Here's how the part is built. I have some questions about the finished solid (model axes, mm). A direction names the side the tool comes from. Round coordinates to 2 decimals unless told otherwise and drop trailing zeros. Order: outer loops, then holes, each group sorted by start corner. A loop starts at its lowest first (then second) coordinate and runs counter-clockwise, first axis right, second up. Notation, with made-up numbers: M 19.25,66.25 L 61.25,66.25 A31 cw 61.25,95.25 Z; hole C -28,-33.75 d8. An arc over 180 degrees is marked long. Write item = value, one per line. Start each with the question number.
Item 1: I'm going to push flat-ended pins straight in: P1, Ø4, axis at x = 10, z = 0, coming from the +Y side; P2, Ø8, axis at x = 11.5, y = -6.5, coming from the -Z side; P3, Ø5, axis at x = 4.5, z = -11, coming from the -Y side. Where does each tip first touch, or does it pass through?
Item 2: For faces 4 (the face through (7, -11, 0)), 5 (the face through (-2, -15, 15)), 6 (the face through (7, 0, 9)), 7 (the face through (7, 0, 11)), 8 (the face through (-3, 0, 0)), which set-ups out of +Z, -Z, +X, -X, +Y, -Y let a thin tool reach every point of the face, with its end or its side?
Item 3: I want a section at A-A, the plane x = 10. List the corners of the cut face in (y, z) for me, plus the area to 3 significant figures.
Item 4: We'd pull the mould along X, two halves only. Please class faces 1 (the face through (7, 0, -11)), 2 (the face through (0, 14, 0)), 3 (the face through (9.63, -9.99, 1.66)): pulls with the +X half, pulls with the -X half, needs draft (parallel to the pull), parting line crosses it, or undercut.
Item 5: I want a section at B-B, the plane z = 16. List the corners of the cut face in (x, y) for me, plus the area to 3 significant figures.
Item 6: I want a section at D-D, the plane y = 0. List the corners of the cut face in (x, z) for me.
Item 7: Please list where these lines run through material, in increasing order: L1, parallel to Z at x = 4.75, y = 6; L2, parallel to Z at x = 10, y = 9.5.
Item 8: I want a section at C-C, the plane x = 5. List the corners of the cut face in (y, z) for me.
Autodesk Inventor part; units mm, degrees
ref_plane "YZ Plane" through (0, 0, 0) normal (1, 0, 0) x (0, 1, 0)
ref_plane "XZ Plane" through (0, 0, 0) normal (0, 1, 0) x (-1, 0, 0)
ref_plane "XY Plane" through (0, 0, 0) normal (0, 0, 1) x (1, 0, 0)
sketch "スケッチ1" plane through (0, 0, 0) normal (1, 0, 0) x (0, 1, 0)
  line L0 (9, -9) -> (-9, -9)
  line L1 (-9, -9) -> (-9, 9)
  line L2 (-9, 9) -> (9, 9)
  line L3 (9, 9) -> (9, -9)
  line L4 (9, -9) -> (-9, 9) construction
  line L5 (-9, -9) -> (9, 9) construction
  line L6 (11, -11) -> (-11, -11)
  line L7 (-11, -11) -> (-11, 11)
  line L8 (-11, 11) -> (11, 11)
  line L9 (11, 11) -> (11, -11)
  line L10 (11, -11) -> (-11, 11) construction
  line L11 (-11, -11) -> (11, 11) construction
  point P0 (0, 0)
  dimension "d0" = 18
  dimension "d1" = 18
  dimension "d2" = 22
  dimension "d3" = 22
extrude "押し出し1" add sketch "スケッチ1" along normal blind 15
sketch "スケッチ2" plane through (0, -11, 11) normal (0, 0, 1) x (1, 0, 0)
  circle A0 centre (10, 11) radius 1.7
  point P0 (0, 11)
  dimension "d6" = 3.4
extrude "押し出し2" cut sketch "スケッチ2" against normal blind 30
sketch "スケッチ3" plane through (0, 11, 11) normal (0, 1, 0) x (1, 0, 0)
  circle A0 centre (10, 11) radius 1.7
  point P0 (0, 11)
  dimension "d9" = 3.4
extrude "押し出し3" cut sketch "スケッチ3" against normal blind 30
sketch "スケッチ4" plane through (0, 0, 0) normal (-1, 0, 0) x (0, 0, 1)
  line L0 (20, -20) -> (-20, -20)
  line L1 (-20, -20) -> (-20, 20)
  line L2 (-20, 20) -> (20, 20)
  line L3 (20, 20) -> (20, -20)
  line L4 (20, -20) -> (-20, 20) construction
  line L5 (-20, -20) -> (20, 20) construction
  point P0 (0, 0)
  dimension "d12" = 40
  dimension "d13" = 40
extrude "押し出し4" add sketch "スケッチ4" along normal blind 3
sketch "スケッチ5" plane through (-3, 0, 0) normal (-1, 0, 0) x (0, 0, 1)
  circle A0 centre (16, 0) radius 2.25
  circle A1 centre (-16, 0) radius 2.25
  point P0 (0, 0)
  dimension "d16" = 4.5
  dimension "d17" = 4.5
extrude "押し出し5" cut sketch "スケッチ5" against normal blind 3
sketch "スケッチ6" plane through (-3, 0, 0) normal (-1, 0, 0) x (0, 0, 1)
  line L0 (20, 20) -> (-20, 20)
  line L1 (10, 20) -> (20, 10)
  line L2 (20, -20) -> (20, 20)
  line L3 (10, 20) -> (24.1421, 20) construction
  line L4 (20, 10) -> (20, 20)
  line L5 (20, 20) -> (10, 20)
  line L6 (-20, -20) -> (20, -20)
  line L7 (20, -20) -> (10, -20)
  line L8 (10, -20) -> (20, -10)
  line L9 (20, -10) -> (20, -20)
  line L10 (-20, 20) -> (-20, -20)
  line L11 (-20, -20) -> (-10, -20)
  line L12 (-10, -20) -> (-20, -10)
  line L13 (-20, -10) -> (-20, -20)
  line L14 (-20, 20) -> (-10, 20)
  line L15 (-10, 20) -> (-20, 10)
  line L16 (-20, 10) -> (-20, 20)
  point P0 (0, 0)
  dimension "d20" = 45
  dimension "d21" = 10
  dimension "d22" = 45
  dimension "d23" = 10
  dimension "d24" = 45
  dimension "d25" = 10
  dimension "d26" = 45
extrude "押し出し6" cut sketch "スケッチ6" against normal blind 3 contours L2 L1 L0 | L15 L10 L0 | L2 L6 L8 | L12 L6 L10
properties part number "square_ber_holder" material "ABS プラスチック"
Filled in:
q1.P1 = 11
q1.P2 = -11
q1.P3 = -11
q2.face_4 = +Z, -Z, +X, -Y
q2.face_5 = +Z, +X, -X, -Y
q2.face_6 = +X
q2.face_7 = +Z, +X, +Y, -Y
q2.face_8 = +Z, -Z, -X, +Y, -Y
q3.outline = M -11,-11 L -1.7,-11 L -1.7,-9 L -9,-9 L -9,-1.7 L -11,-1.7 Z; M -11,1.7 L -9,1.7 L -9,9 L -1.7,9 L -1.7,11 L -11,11 Z; M 1.7,-11 L 11,-11 L 11,-1.7 L 9,-1.7 L 9,-9 L 1.7,-9 Z; M 1.7,9 L 9,9 L 9,1.7 L 11,1.7 L 11,11 L 1.7,11 Z
q3.area = 133 mm^2
q4.face_1 = needs draft
q4.face_2 = pulls with the +X half
q4.face_3 = undercut
q5.outline = M -3,-14 L 0,-14 L 0,-2.25 L -3,-2.25 Z; M -3,2.25 L 0,2.25 L 0,14 L -3,14 Z
q5.area = 70.5 mm^2
q6.outline = M -3,-20 L 0,-20 L 0,-18.25 L -3,-18.25 Z; M -3,-13.75 L 0,-13.75 L 0,-11 L 8.3,-11 L 8.3,-9 L 0,-9 L 0,9 L 8.3,9 L 8.3,11 L 0,11 L 0,13.75 L -3,13.75 Z; M -3,18.25 L 0,18.25 L 0,20 L -3,20 Z; M 11.7,-11 L 15,-11 L 15,-9 L 11.7,-9 Z; M 11.7,9 L 15,9 L 15,11 L 11.7,11 Z
q7.L1 = -11 to -9, 9 to 11
q7.L2 = -11 to -1.7, 1.7 to 11
q8.outline = M -11,-11 L 11,-11 L 11,11 L -11,11 Z; hole M -9,-9 L 9,-9 L 9,9 L -9,9 Z
